The listing builds one solid part. Answer for the finished solid, in the listing's coordinates (mm). Coordinates: 2 decimals unless noted, no trailing zeros. Order: outer loops, then holes, each group sorted by start corner. A loop starts at its lowest first (then second) coordinate and runs counter-clockwise, first axis right, second up. Notation, with made-up numbers: (44, 84.25) -> (51, 84.25) arc R18 cw to (51, 117.25) -> close; hole circle Ø5 at (58.5, 67). An arc over 180 degrees is marked (long way). Answer in a Markdown table with one row per item.
```python
from build123d import *

# Parameters (mm, degrees)
SHEET_EXTRUDE_DEPTH      = 31.8
M3_CLEARANCE_HOLE1_D     = 3.4
M3_CLEARANCE_HOLE1_DEPTH = 8.5
M3_CLEARANCE_HOLE1_TIP   = 1.021463052
M4_CLEARANCE_HOLE1_D     = 4.5
M4_CLEARANCE_HOLE1_DEPTH = 8.5
M4_CLEARANCE_HOLE1_TIP   = 1.351936393
FILLET1_R                = 10


with BuildPart() as part:
    # Sketch2 → Sheet Extrude (new body, symmetric)
    with BuildSketch(Plane(origin=(0, 0, 0), x_dir=(0, 0, -1), z_dir=(1, 0, 0))):
        Polygon((0, 0), (0, 2), (-35, 2), (-55, 2), (-115, 2), (-115, 0), (-55, 0), (-35, 0), align=None)
    extrude(amount=SHEET_EXTRUDE_DEPTH, both=True)

    # M3 Clearance Hole1
    with Locations(Plane(origin=(0, 2, 0), x_dir=(1, 0, 0), z_dir=(0, 1, 0))):
        with Locations((-22, -108), (-22, -85), (-8, -85), (-8, -108), (22, -108), (8, -108), (8, -85), (22, -85)):
            Hole(M3_CLEARANCE_HOLE1_D / 2, depth=M3_CLEARANCE_HOLE1_DEPTH)
            with Locations((0, 0, -(M3_CLEARANCE_HOLE1_DEPTH + M3_CLEARANCE_HOLE1_TIP / 2))):  # 118° drill point
                Cone(0, M3_CLEARANCE_HOLE1_D / 2, M3_CLEARANCE_HOLE1_TIP, mode=Mode.SUBTRACT)

    # M4 Clearance Hole1
    with Locations(Plane(origin=(0, 2, 0), x_dir=(1, 0, 0), z_dir=(0, 1, 0))):
        with Locations((-20, -28), (20, -28), (20, -8), (-20, -8)):
            Hole(M4_CLEARANCE_HOLE1_D / 2, depth=M4_CLEARANCE_HOLE1_DEPTH)
            with Locations((0, 0, -(M4_CLEARANCE_HOLE1_DEPTH + M4_CLEARANCE_HOLE1_TIP / 2))):  # 118° drill point
                Cone(0, M4_CLEARANCE_HOLE1_D / 2, M4_CLEARANCE_HOLE1_TIP, mode=Mode.SUBTRACT)

    # Fillet1
    fillet1_edges = [part.edges().sort_by_distance(p)[0] for p in [
        (-31.8, 1, 0),
        (31.8, 1, 0),
    ]]
    fillet(fillet1_edges, radius=FILLET1_R)


solid = part.part
```
(1) A cutting plane is placed at B-B, the plane z = 85. Determine the outline of the cut face in (x, y).
Check values:
| item | result |
|---|---|
| outline | (-31.8, 0) -> (-23.7, 0) -> (-23.7, 2) -> (-31.8, 2) -> close; (-20.3, 0) -> (-9.7, 0) -> (-9.7, 2) -> (-20.3, 2) -> close; (-6.3, 0) -> (6.3, 0) -> (6.3, 2) -> (-6.3, 2) -> close; (9.7, 0) -> (20.3, 0) -> (20.3, 2) -> (9.7, 2) -> close; (23.7, 0) -> (31.8, 0) -> (31.8, 2) -> (23.7, 2) -> close |
(2) For a pull along Z with two mould halves and no side action, classify faces 1 (the flat face through (0, 0, 58)), 2 (the cylindrical face through (17.854, 0.986, 7.324)), 3 (the cylindrical face through (-28.79, 1.01, 2.85)) as released by +Z, released by -Z, zero draft, split by the parting line, or undercut.
Check values:
| item | result |
|---|---|
| face 1 | zero draft |
| face 2 | undercut |
| face 3 | released by -Z |
(3) Flat-ended cylindrical pins translate along their axes: pin 1 (2.5 mm diameter, centred on x = 22, z = 85, fed in from -Y); pin 2 (4.5 mm diameter, centred on x = 8, z = 108, fed in from +Y). Find the tip coordinate at first contact, or state that the pin passes through.
Check values:
| item | result |
|---|---|
| pin 1 | through |
| pin 2 | y = 2 |
(4) A cutting plane is placed at D-D, the plane y = 1.4. Count the separate pieces of the cut face and the enclosed holes in it, then the cut area to 3 significant figures.
Check values:
| item | result |
|---|---|
| separate pieces | 1 |
| enclosed holes | 12 |
| area | 7,130 mm² |
(5) Find the intervals of material crossed by line 1 along X through (y, z) = (1.45, 85); line 2 along Z through (x, y) = (-8, 1.15); line 3 along Z through (x, y) = (-20, 0.7), in increasing order. Write a range as from..to.
Check values:
| item | result |
|---|---|
| line 1 | -31.8..-23.7, -20.3..-9.7, -6.3..6.3, 9.7..20.3, 23.7..31.8 |
| line 2 | 0..83.3, 86.7..106.3, 109.7..115 |
| line 3 | 0..5.75, 10.25..25.75, 30.25..115 |
(6) A cutting plane is placed at A-A, the plane x = -8. Determine the outline of the cut face in (y, z), then the cut area to 3 significant figures.
Check values:
| item | result |
|---|---|
| outline | (0, 0) -> (2, 0) -> (2, 83.3) -> (0, 83.3) -> close; (0, 86.7) -> (2, 86.7) -> (2, 106.3) -> (0, 106.3) -> close; (0, 109.7) -> (2, 109.7) -> (2, 115) -> (0, 115) -> close |
| area | 216 mm² |
(7) A cutting plane is placed at C-C, the plane z = 28. Determine the outline of the cut face in (x, y), then the cut area to 3 significant figures.
Check values:
| item | result |
|---|---|
| outline | (-31.8, 0) -> (-22.25, 0) -> (-22.25, 2) -> (-31.8, 2) -> close; (-17.75, 0) -> (17.75, 0) -> (17.75, 2) -> (-17.75, 2) -> close; (22.25, 0) -> (31.8, 0) -> (31.8, 2) -> (22.25, 2) -> close |
| area | 109 mm² |
